Source: CAD feature listing. Evaluate the final solid. Frame: model axes, mm. A direction names the side the tool comes from. Round coordinates to 2 decimals unless told otherwise and drop trailing zeros. Loops run counter-clockwise (first coordinate to the right, second up) from the corner with the lowest first, then second, coordinate; pieces in that order, holes last. Notation, with made-up numbers: (-22.5, 3.25) - (24.5, 3.25) arc R22 cw to (24.5, 25.25) - close; hole circle Ø8 at (62.5, -27.75). An arc over 180 degrees is marked (long way). Write item = value, one per line. Start each with the question number.
from build123d import *

# Parameters (mm, degrees)
SKETCH009_R             = 1.9
PAD006_DEPTH            = 3
SKETCH010_W             = 18
SKETCH010_H             = 18
SKETCH010_R             = 1.9
PAD007_DEPTH            = 3
SKETCH011_W             = 18
SKETCH011_H             = 18
SKETCH011_R             = 1.9
PAD008_DEPTH            = 3
BODY008_PLACEMENT_ANGLE = 180


with BuildPart() as part:
    # Sketch009 → Pad006 (new body)
    with BuildSketch(Plane.XY):
        Polygon((0, -18), (0, 0), (18, 0), (18, -6), (6, -18), align=None)
        with Locations((6, -12)):
            Circle(SKETCH009_R, mode=Mode.SUBTRACT)
        with Locations((12, -6)):
            Circle(SKETCH009_R, mode=Mode.SUBTRACT)
    extrude(amount=PAD006_DEPTH)

    # Sketch010 (on Face1 of Pad006) → Pad007 (join)
    with BuildSketch(Plane(origin=(3, 0, 0), x_dir=(0, -1, 0), z_dir=(-1, 0, 0))):
        with Locations((9, 9)):
            Rectangle(SKETCH010_W, SKETCH010_H)
        with Locations((9, 14)):
            Circle(SKETCH010_R, mode=Mode.SUBTRACT)
    extrude(amount=PAD007_DEPTH)

    # Sketch011 (on Face2 of Pad006) → Pad008 (join)
    with BuildSketch(Plane(origin=(0, 0, 0), x_dir=(-1, 0, 0), z_dir=(0, 1, 0))):
        with Locations((-9, 9)):
            Rectangle(SKETCH011_W, SKETCH011_H)
        with Locations((-9, 14)):
            Circle(SKETCH011_R, mode=Mode.SUBTRACT)
    extrude(amount=-PAD008_DEPTH)


with BuildPart() as part_1:
    # Body005 placement: moved
    add(part.part.moved(Location((25, 0, 3.3))))


with BuildPart() as part_2:
    # Body008 placement: moved
    add(part_1.part.moved(Location((226, -81.5, 0))).rotate(Axis((226, -81.5, 0), (0, 0, 1)), BODY008_PLACEMENT_ANGLE))


solid = part_2.part
(1) Cut plane D-D (y = -66.75). Output: boundary loops of the cut face in (x, z), and give its area (4 significant figures).
(2) Cut plane B-B (y = -69.5). Output: boundary loops of the cut face in (x, z), and give its area (3 significant figures).
(3) Cut plane C-C (x = 198.25). Output: boundary loops of the cut face in (y, z), and give its area (3 significant figures).
(4) Cut plane A-A (x = 192). Output: boundary loops of the cut face in (y, z), and give its area (3 significant figures).
(5) Mould query, pull axis Y, two halves, no side actions, for faces 1 (the face through (192, -81.5, 12)), 2 (the face through (192, -73, 6.3)), 3 (the face through (188.9, -69.6, 4.8)), 4 (the face through (195.412, -67.645, 4.779)). Classes: +Y half, -Y half, draft (parallel to the pull), parting line (faces both ways), or undercut.
(6) Access query for faces 5 (the face through (190.1, -80.02, 17.38)), 6 (the face through (198, -71, 14)). Directions: +Z, -Z, +X, -X, +Y, -Y. A direction counts if a zero-diameter tool reaches every point of the face in a straight line with its end or side. Return the directions, or none.
(7) Material intervals for line 1 along Y through (x, z) = (185.75, 19); line 2 along X through (y, z) = (-74, 9.5); line 3 along Z through (x, y) = (184, -77.25), sorted ascending. Write a range as from..to.
(8) Pin query (flat end, axial travel): P1, Ø5, axis at y = -72.5, z = 17.3, coming from the -X side; P2, Ø8, axis at x = 191.5, z = 15.5, coming from the +Y side; P3, Ø2.5, axis at x = 192, z = 17.3, coming from the +Y side. Return the tip coordinate at first contact, or that it passes through.
Solution:
q1.outline = (191.75, 3.3) - (201, 3.3) - (201, 21.3) - (198, 21.3) - (198, 6.3) - (191.75, 6.3) - close
q1.area = 72.75 mm^2
q2.outline = (189, 3.3) - (193.1, 3.3) - (193.1, 6.3) - (189, 6.3) - close; (196.9, 3.3) - (201, 3.3) - (201, 21.3) - (198, 21.3) - (198, 6.3) - (196.9, 6.3) - close
q2.area = 69.6 mm^2
q3.outline = (-81.5, 3.3) - (-63.5, 3.3) - (-63.5, 21.3) - (-81.5, 21.3) - close; hole circle Ø3.8 at (-72.5, 17.3)
q3.area = 313 mm^2
q4.outline = (-81.5, 3.3) - (-66.5, 3.3) - (-66.5, 6.3) - (-78.5, 6.3) - (-78.5, 15.4) - (-81.5, 15.4) - close; (-81.5, 19.2) - (-78.5, 19.2) - (-78.5, 21.3) - (-81.5, 21.3) - close
q4.area = 78.6 mm^2
q5.face_1 = -Y half
q5.face_2 = draft
q5.face_3 = +Y half
q5.face_4 = undercut
q6.face_5 = +Y, -Y
q6.face_6 = +Z, -X, +Y
q7.line_1 = -81.5..-78.5
q7.line_2 = 198..201
q7.line_3 = 3.3..6.3
q8.P1 = 198
q8.P2 = -78.5
q8.P3 = through
